```python
from build123d import *

# Parameters (mm, degrees)
ESQUISSE1_W             = 60
ESQUISSE1_H             = 40
BOSS_EXTRU_1_DEPTH      = 2
ESQUISSE2_W             = 55
ESQUISSE2_H             = 35
BOSS_EXTRU_2_DEPTH      = 10
CONG_1_R                = 3
CONG_2_R                = 1
ESQUISSE3_W             = 47
ESQUISSE3_H             = 27
ENL_V_MAT_EXTRU_1_DEPTH = 10
ESQUISSE4_R             = 1.5
ENL_V_MAT_EXTRU_2_DEPTH = 72.765242283
ESQUISSE5_R             = 11.1
ESQUISSE5_R_2           = 1.2
ENL_V_MAT_EXTRU_3_DEPTH = 74.10266753
ESQUISSE6_R             = 2.75
ENL_V_MAT_EXTRU_4_DEPTH = 73.801098893


with BuildPart() as part:
    # Esquisse1 → Boss.-Extru.1 (new body)
    with BuildSketch(Plane.XY):
        with Locations((30, 20)):
            Rectangle(ESQUISSE1_W, ESQUISSE1_H)
    extrude(amount=BOSS_EXTRU_1_DEPTH)

    # Esquisse2 → Boss.-Extru.2 (add)
    with BuildSketch(Plane.XY.offset(2)):
        with Locations((30, 20)):
            Rectangle(ESQUISSE2_W, ESQUISSE2_H)
    extrude(amount=BOSS_EXTRU_2_DEPTH)

    # Congé1
    cong_1_edges = [part.edges().sort_by_distance(p)[0] for p in [
        (57.5, 37.5, 7),
        (2.5, 37.5, 7),
        (2.5, 2.5, 7),
        (57.5, 2.5, 7),
    ]]
    fillet(cong_1_edges, radius=CONG_1_R)

    # Congé2
    cong_2_edges = [part.edges().sort_by_distance(p)[0] for p in [
        (0, 40, 1),
        (60, 40, 1),
        (60, 0, 1),
        (0, 0, 1),
    ]]
    fillet(cong_2_edges, radius=CONG_2_R)

    # Esquisse3 → Enlèv. mat.-Extru.1 (cut)
    with BuildSketch(Plane.XY.offset(12)):
        with Locations((30, 20)):
            Rectangle(ESQUISSE3_W, ESQUISSE3_H)
    extrude(amount=-ENL_V_MAT_EXTRU_1_DEPTH, mode=Mode.SUBTRACT)

    # Esquisse4 → Enlèv. mat.-Extru.2 (cut, through all)
    with BuildSketch(Plane(origin=(0, 37.5, 0), x_dir=(1, 0, 0), z_dir=(0, 1, 0))):
        with Locations(Location((30, -7, 0), (0, 0, 270))):
            Circle(ESQUISSE4_R)
    extrude(amount=-ENL_V_MAT_EXTRU_2_DEPTH, mode=Mode.SUBTRACT)

    # Esquisse5 → Enlèv. mat.-Extru.3 (cut, through all)
    with BuildSketch(Plane(origin=(0, 0, 0), x_dir=(-1, 0, 0), z_dir=(0, 0, -1))):
        with Locations((-42.5, 20)):
            Circle(ESQUISSE5_R)
        with Locations((-17.5, 20)):
            Circle(ESQUISSE5_R)
        with Locations((-52.4, 29.9)):
            Circle(ESQUISSE5_R_2)
        with Locations((-32.6, 10.1)):
            Circle(ESQUISSE5_R_2)
        with Locations((-27.4, 29.9)):
            Circle(ESQUISSE5_R_2)
        with Locations((-7.6, 10.1)):
            Circle(ESQUISSE5_R_2)
    extrude(amount=-ENL_V_MAT_EXTRU_3_DEPTH, mode=Mode.SUBTRACT)

    # Esquisse6 → Enlèv. mat.-Extru.4 (cut, through all)
    with BuildSketch(Plane.XY.offset(2)):
        with Locations((7.6, 10.1)):
            Circle(ESQUISSE6_R)
        with Locations((52.4, 29.9)):
            Circle(ESQUISSE6_R)
    extrude(amount=ENL_V_MAT_EXTRU_4_DEPTH, mode=Mode.SUBTRACT)


solid = part.part
```
Check sheet for the modelled part. Datum: model origin and axes. Units: mm. A direction names the side the tool comes from. Give positions to 0.01 mm unless a question says otherwise; leave off trailing zeros. Loops run counter-clockwise (first coordinate to the right, second up) from the corner with the lowest first, then second, coordinate; pieces in that order, holes last. Notation, with made-up numbers: M 63,-34.75 L 72,-34.75 A13 cw 72,-18.75 Z; hole C -36.75,63.5 d7. An arc over 180 degrees is marked long. Answer in a Markdown table with one row per item.
1) Tool access check on faces 4 (the face through (8.8, 10.15, 0.99)), 5 (the face through (3.4, 36.64, 7.07)), 6 (the face through (2.5, 20, 7)), 7 (the face through (53.5, 24, 7)). Record the directions out of +Z, -Z, +X, -X, +Y, -Y that give a thin tool (end or side, any length) a straight path to the whole face; none if there is none.
Solutions:
| item | result |
|---|---|
| face 4 | +Z, -Z |
| face 5 | +Z, -X, +Y |
| face 6 | +Z, -X, +Y, -Y |
| face 7 | +Z |
2) Cross-section at A-A (x = 17.5). Enter the section's corners in (y, z), plus the area to 3 significant figures.
Solutions:
| item | result |
|---|---|
| outline | M 0,0 L 8.9,0 L 8.9,2 L 6.5,2 L 6.5,12 L 2.5,12 L 2.5,2 L 0,2 Z; M 31.1,0 L 40,0 L 40,2 L 37.5,2 L 37.5,12 L 33.5,12 L 33.5,2 L 31.1,2 Z |
| area | 116 mm^2 |
3) Mould release check, pull along Y, two halves, no side actions. Record for faces 1 (the face through (53.5, 12, 7)), 2 (the face through (56.6, 3.36, 7.07)), 3 (the face through (30, 37.5, 5)): released by +Y, released by -Y, zero draft, split by the parting line, or undercut.
Solutions:
| item | result |
|---|---|
| face 1 | undercut |
| face 2 | released by -Y |
| face 3 | released by +Y |
4) Cross-section at C-C (y = 20). Enter the section's corners in (x, z).
Solutions:
| item | result |
|---|---|
| outline | M 0,0 L 6.4,0 L 6.4,12 L 2.5,12 L 2.5,2 L 0,2 Z; M 28.6,0 L 31.4,0 L 31.4,2 L 28.6,2 Z; M 53.6,0 L 60,0 L 60,2 L 57.5,2 L 57.5,12 L 53.6,12 Z |
5) Cross-section at D-D (z = 1). Enter the section's corners in (x, y), plus the area to 3 significant figures.
Solutions:
| item | result |
|---|---|
| outline | M 0,1 A1 ccw 1,0 L 59,0 A1 ccw 60,1 L 60,39 A1 ccw 59,40 L 1,40 A1 ccw 0,39 Z; hole C 7.6,10.1 d2.4; hole C 17.5,20 d22.2; hole C 27.4,29.9 d2.4; hole C 32.6,10.1 d2.4; hole C 42.5,20 d22.2; hole C 52.4,29.9 d2.4 |
| area | 1,610 mm^2 |
6) Thickness scan on line 1 (Y direction, x = 24, z = 2.75); line 2 (X direction, y = 17.5, z = 4.5); line 3 (X direction, y = 20, z = 9). Record the ranges inside material, lowest first.
Solutions:
| item | result |
|---|---|
| line 1 | y = 2.5 to 6.5, 33.5 to 37.5 |
| line 2 | x = 2.5 to 6.5, 53.5 to 57.5 |
| line 3 | x = 2.5 to 6.4, 53.6 to 57.5 |
7) Depth check by flat-ended pin: pin 1 (3 mm diameter, centred on x = 32.6, y = 10.1, fed in from -Z); pin 2 (2.5 mm diameter, centred on x = 30, z = 7, fed in from +Y); pin 3 (1.5 mm diameter, centred on y = 17, z = 7, fed in from -X); pin 4 (5 mm diameter, centred on x = 41, z = 6, fed in from +Y). Enter the tip coordinate at first touch or a pass-through.
Solutions:
| item | result |
|---|---|
| pin 1 | stops at z = 0 |
| pin 2 | passes through |
| pin 3 | stops at x = 2.5 |
| pin 4 | stops at y = 37.5 |
8) Cross-section at B-B (z = 7). Enter the section's corners in (x, y), plus the area to 3 significant figures.
Solutions:
| item | result |
|---|---|
| outline | M 2.5,5.5 A3 ccw 5.5,2.5 L 28.5,2.5 L 28.5,6.5 L 6.5,6.5 L 6.5,7.58 A2.75 cw 6.5,12.62 L 6.5,18.51 A11.1 cw 6.5,21.49 L 6.5,33.5 L 28.5,33.5 L 28.5,37.5 L 5.5,37.5 A3 ccw 2.5,34.5 Z; M 31.5,2.5 L 54.5,2.5 A3 ccw 57.5,5.5 L 57.5,34.5 A3 ccw 54.5,37.5 L 31.5,37.5 L 31.5,33.5 L 53.5,33.5 L 53.5,32.42 A2.75 cw 53.5,27.38 L 53.5,21.49 A11.1 cw 53.5,18.51 L 53.5,6.5 L 31.5,6.5 Z |
| area | 612 mm^2 |
